from build123d import *

# Parameters (mm, degrees)
SKETCH1_R           = 1.6
BOSS_EXTRUDE1_DEPTH = 8
CHAMFER1_SIZE       = 1
SKETCH2_R           = 1.6
BOSS_EXTRUDE3_DEPTH = 8
FILLET1_R           = 10
CHAMFER2_SIZE       = 1
CHAMFER3_SIZE       = 1
CHAMFER4_SIZE       = 1


with BuildPart() as part:
    # Sketch1 → Boss-Extrude1 (new body)
    with BuildSketch(Plane.XY):
        with BuildLine():
            Line((-0.5, 3), (60.5, 3))
            ThreePointArc((60.5, 3), (62.267766953, 2.267766953), (63, 0.5))
            Line((63, 0.5), (63, -0.5))
            ThreePointArc((63, -0.5), (62.267766953, -2.267766953), (60.5, -3))
            Line((60.5, -3), (-0.5, -3))
            ThreePointArc((-0.5, -3), (-2.267766953, -2.267766953), (-3, -0.5))
            Line((-3, -0.5), (-3, 0.5))
            ThreePointArc((-3, 0.5), (-2.267766953, 2.267766953), (-0.5, 3))
        make_face()
        Circle(SKETCH1_R, mode=Mode.SUBTRACT)
        with Locations((7.5, 0)):
            Circle(SKETCH1_R, mode=Mode.SUBTRACT)
        with Locations((15, 0)):
            Circle(SKETCH1_R, mode=Mode.SUBTRACT)
        with Locations((22.5, 0)):
            Circle(SKETCH1_R, mode=Mode.SUBTRACT)
        with Locations((30, 0)):
            Circle(SKETCH1_R, mode=Mode.SUBTRACT)
        with Locations((37.5, 0)):
            Circle(SKETCH1_R, mode=Mode.SUBTRACT)
        with Locations((45, 0)):
            Circle(SKETCH1_R, mode=Mode.SUBTRACT)
        with Locations((52.5, 0)):
            Circle(SKETCH1_R, mode=Mode.SUBTRACT)
        with Locations((60, 0)):
            Circle(SKETCH1_R, mode=Mode.SUBTRACT)
    extrude(amount=BOSS_EXTRUDE1_DEPTH)

    # Chamfer1
    chamfer1_edges = [part.edges().sort_by_distance(p)[0] for p in [
        (-1.6, 0, 0),
        (-1.6, 0, 8),
        (5.9, 0, 0),
        (5.9, 0, 8),
        (13.4, 0, 0),
        (13.4, 0, 8),
        (20.9, 0, 0),
        (20.9, 0, 8),
        (28.4, 0, 0),
        (28.4, 0, 8),
    ]]
    chamfer(chamfer1_edges, length=CHAMFER1_SIZE)

    # Sketch2 → Boss-Extrude3 (add)
    with BuildSketch(Plane.XY.offset(8)):
        with BuildLine():
            ThreePointArc((-3, 0.5), (-2.809698831, 1.456708581), (-2.267766953, 2.267766953))
            Line((-2.267766953, 2.267766953), (-18.529200529, -13.993666623))
            ThreePointArc((-18.529200529, -13.993666623), (-19.261433576, -15.761433576), (-18.529200529, -17.529200529))
            Line((-18.529200529, -17.529200529), (-17.822093748, -18.23630731))
            ThreePointArc((-17.822093748, -18.23630731), (-16.054326795, -18.968540357), (-14.286559842, -18.23630731))
            Line((-14.286559842, -18.23630731), (0.949747468, -3))
            Line((0.949747468, -3), (-0.5, -3))
            ThreePointArc((-0.5, -3), (-2.267766953, -2.267766953), (-3, -0.5))
            Line((-3, -0.5), (-3, 0.5))
        make_face()
        with Locations((-16.054326795, -15.761433576)):
            Circle(SKETCH2_R, mode=Mode.SUBTRACT)
        with Locations((-10.751025936, -10.458132717)):
            Circle(SKETCH2_R, mode=Mode.SUBTRACT)
        with Locations((-5.447725077, -5.154831858)):
            Circle(SKETCH2_R, mode=Mode.SUBTRACT)
    extrude(amount=-BOSS_EXTRUDE3_DEPTH)

    # Fillet1
    fillet1_edges = [part.edges().sort_by_distance(p)[0] for p in [
        (0.949747468, -3, 4),
    ]]
    fillet(fillet1_edges, radius=FILLET1_R)

    # Chamfer2
    chamfer2_edges = [part.edges().sort_by_distance(p)[0] for p in [
        (-17.654326795, -15.761433576, 0),
        (-17.654326795, -15.761433576, 8),
        (-12.351025936, -10.458132717, 8),
        (-7.047725077, -5.154831858, 8),
        (-7.047725077, -5.154831858, 0),
        (-12.351025936, -10.458132717, 0),
    ]]
    chamfer(chamfer2_edges, length=CHAMFER2_SIZE)

    # Chamfer3
    chamfer3_edges = [part.edges().sort_by_distance(p)[0] for p in [
        (35.9, 0, 0),
        (35.9, 0, 8),
        (43.4, 0, 0),
        (43.4, 0, 8),
    ]]
    chamfer(chamfer3_edges, length=CHAMFER3_SIZE)

    # Chamfer4
    chamfer4_edges = [part.edges().sort_by_distance(p)[0] for p in [
        (50.9, 0, 0),
        (50.9, 0, 8),
        (58.4, 0, 0),
        (58.4, 0, 8),
    ]]
    chamfer(chamfer4_edges, length=CHAMFER4_SIZE)


solid = part.part
Geometry check sheet. Reference: the model listing, model coordinates, mm. Give positions to 0.01 mm unless a question says otherwise; leave off trailing zeros. Write each loop counter-clockwise with the first axis right and the second up, starting at its lowest first coordinate (ties: lowest second). Pieces come first, ordered by that corner, then holes. Notation, with made-up numbers: (50.25, 89) - (83.25, 89) arc R14 cw to (83.25, 113) - close; hole circle Ø7 at (9.25, 56). An arc over 180 degrees is marked (long way). Put each result on its own line as item: value.
1. Sectioned sample at B-B, the plane z = 5.25. Give the number of separate pieces and of enclosed holes in the cut face, plus the area to 3 significant figures.
Ans:
separate pieces: 1
enclosed holes: 12
area: 432 mm²
2. Sectioned sample at A-A, the plane x = 45. Enter the section's corners in (y, z), plus the area to 3 significant figures.
Ans:
outline: (-3, 0) - (-2.6, 0) - (-1.6, 1) - (-1.6, 7) - (-2.6, 8) - (-3, 8) - close; (1.6, 1) - (2.6, 0) - (3, 0) - (3, 8) - (2.6, 8) - (1.6, 7) - close
area: 20.4 mm²
3. Thickness scan on line 1 (Y direction, x = 30, z = 2.45); line 2 (X direction, y = -16, z = 6.25); line 3 (Y direction, x = 30.5, z = 0.75). Record the ranges inside material, lowest first.
Ans:
line 1: y = -3 to -1.6, 1.6 to 3
line 2: x = -19.25 to -17.64, -14.47 to -12.05
line 3: y = -3 to -1.78, 1.78 to 3
4. Draft check along X on faces 1 (the flat face through (-8.22, -12.17, 4.06)), 2 (the cylindrical face through (-16.08, -18.97, 4.06)), 3 (the cylindrical face through (5.9, 0.07, 3.96)). Enter one of: +X half, -X half, draft (parallel to the pull), parting line (faces both ways), or undercut.
Ans:
face 1: +X half
face 2: parting line
face 3: undercut
5. Go/stop test with flat-tipped pins: pin 1 (5 mm diameter, centred on x = 37.5, y = 0, fed in from +Z); pin 2 (8 mm diameter, centred on x = 31, y = -8, fed in from -Z); pin 3 (3.5 mm diameter, centred on x = -5.45, y = -5.15, fed in from +Z); pin 4 (5 mm diameter, centred on x = 30, y = 0, fed in from -Z). Record where each tip stops, or that it passes through.
Ans:
pin 1: stops at z = 7.9
pin 2: passes through
pin 3: stops at z = 7.16
pin 4: stops at z = 0.1
